Input: part model. Units: mm. Frame: model coordinates. A direction names the side the tool comes from. Coordinates: 2 decimals unless noted, no trailing zeros. Loops run counter-clockwise (first coordinate to the right, second up) from the corner with the lowest first, then second, coordinate; pieces in that order, holes last. Notation, with made-up numbers: M 21,47 L 26,47 A30 cw 26,74 Z; hole C 6.5,51 d11. An arc over 180 degrees is marked long. Use a Markdown table: item, result. Add a question column.
1. Pin query (flat end, axial travel): pin 1 (3 mm diameter, centred on x = 2.5, y = 2, fed in from -Z); pin 2 (2.5 mm diameter, centred on x = 0, y = 0, fed in from -Z); pin 3 (3.5 mm diameter, centred on y = -0.5, z = 13, fed in from +X); pin 4 (8 mm diameter, centred on x = -1.5, y = -20.5, fed in from -Z). Return the tip coordinate at first contact, or that it passes through.
2. Draft query along X for faces 5 (the cylindrical face through (0.29, 2.23, 3.38)), 6 (the flat face through (0, -6, 0)), 7 (the flat face through (-40, 1, -23)). Return one class per face: +X half, -X half, draft (parallel to the pull), parting line (faces both ways), or undercut.
3. Line query: L1, parallel to Y at x = 0, z = 3; L2, parallel to Y at x = -31.5, z = -24; L3, parallel to Y at x = 0, z = 1. Output: solid intervals per line, ascending. Write a range as [from, to].
4. Section C-C on y = 15.5. Output: boundary loops of the cut face in (x, z).
5. Section A-A on x = 0. Output: boundary loops of the cut face in (y, z), then the cut area to 3 significant figures.
6. Section D-D on y = 0. Output: boundary loops of the cut face in (x, z).
7. Section B-B on z = -21. Output: boundary loops of the cut face in (x, y).
8. Set-up query: faces 1 (the flat face through (-15, 4.913, 12)), 2 (the flat face through (-10, -5, 12)), 3 (the cylindrical face through (1.08, -4.88, 0.89)), 4 (the cylindrical face through (-37.47, 7.28, -51.98)). Return all of +Z, -Z, +X, -X, +Y, -Y with unobstructed straight access to the full face (end or side cutting, diameter ignored); none if empty.
```python
from build123d import *

# Parameters (mm, degrees)
SKETCH1_R           = 14
BOSS_EXTRUDE1_DEPTH = 10
SKETCH2_R           = 2.25
CUT_EXTRUDE1_DEPTH  = 5
SKETCH3_R           = 5
CUT_EXTRUDE2_DEPTH  = 1.8
SKETCH4_W           = 10
SKETCH4_H           = 10
BOSS_EXTRUDE2_DEPTH = 8
SKETCH6_W           = 8
SKETCH6_H           = 9.912865289
BOSS_EXTRUDE3_DEPTH = 20
CUT_EXTRUDE3_DEPTH  = 30
SKETCH8_R           = 38
BOSS_EXTRUDE4_DEPTH = 10
SKETCH9_R           = 29
BOSS_EXTRUDE5_DEPTH = 5


with BuildPart() as part:
    # Sketch1 → Boss-Extrude1 (new body)
    with BuildSketch(Plane.XY):
        Circle(SKETCH1_R)
    extrude(amount=BOSS_EXTRUDE1_DEPTH)

    # Sketch2 → Cut-Extrude1 (cut)
    with BuildSketch(Plane(origin=(0, 0, 0), x_dir=(-1, 0, 0), z_dir=(0, 0, -1))):
        Circle(SKETCH2_R)
    extrude(amount=-CUT_EXTRUDE1_DEPTH, mode=Mode.SUBTRACT)

    # Sketch3 → Cut-Extrude2 (cut)
    with BuildSketch(Plane(origin=(0, 0, 0), x_dir=(-1, 0, 0), z_dir=(0, 0, -1))):
        Circle(SKETCH3_R)
    extrude(amount=-CUT_EXTRUDE2_DEPTH, mode=Mode.SUBTRACT)

    # Sketch4 → Boss-Extrude2 (add)
    with BuildSketch(Plane.XY.offset(10)):
        Rectangle(SKETCH4_W, SKETCH4_H)
    extrude(amount=BOSS_EXTRUDE2_DEPTH)

    # Sketch6 → Boss-Extrude3 (add)
    with BuildSketch(Plane.ZY.offset(5)):
        with Locations((14, -0.043567356)):
            Rectangle(SKETCH6_W, SKETCH6_H)
    extrude(amount=BOSS_EXTRUDE3_DEPTH)

    # Sketch7 → Cut-Extrude3 (cut)
    with BuildSketch(Plane(origin=(5, 0, 0), x_dir=(0, 0, -1), z_dir=(1, 0, 0))):
        with BuildLine():
            Line((-18, 5), (-18, -5))
            Line((-18, -5), (-14, -5))
            ThreePointArc((-14, -5), (-14.330383596, 0), (-14, 5))
            Line((-14, 5), (-18, 5))
        make_face()
    extrude(amount=-CUT_EXTRUDE3_DEPTH, mode=Mode.SUBTRACT)

    # Sketch8 → Boss-Extrude4 (add)
    with BuildSketch(Plane.ZY.offset(25)):
        with Locations(Location((-23.669616404, 0, 0), (0, 0, 7.560843177))):
            Circle(SKETCH8_R)
    extrude(amount=BOSS_EXTRUDE4_DEPTH)

    # Sketch9 → Boss-Extrude5 (add)
    with BuildSketch(Plane.ZY.offset(35)):
        with Locations(Location((-23.669616404, 0.99287457, 0), (0, 0, 270))):
            Circle(SKETCH9_R)
    extrude(amount=BOSS_EXTRUDE5_DEPTH)


solid = part.part
```
Answers below:
| question | item | result |
|---|---|---|
| 1 | pin 1 | stops at z = 1.8 |
| 1 | pin 2 | stops at z = 5 |
| 1 | pin 3 | stops at x = 5 |
| 1 | pin 4 | passes through |
| 2 | face 5 | undercut |
| 2 | face 6 | draft |
| 2 | face 7 | -X half |
| 3 | L1 | y = [-14, -2.25], [2.25, 14] |
| 3 | L2 | y = [-38, 38] |
| 3 | L3 | y = [-14, -5], [5, 14] |
| 4 | outline | M -40,-48.78 L -35,-48.78 L -35,-58.36 L -25,-58.36 L -25,11.03 L -35,11.03 L -35,1.44 L -40,1.44 Z |
| 5 | outline | M -14,0 L -5,0 L -5,1.8 L -2.25,1.8 L -2.25,5 L 2.25,5 L 2.25,1.8 L 5,1.8 L 5,0 L 14,0 L 14,10 L 5,10 L 5,14 A38 ccw -5,14 L -5,10 L -14,10 Z |
| 5 | area | 290 mm² |
| 6 | outline | M -40,-52.65 L -35,-52.65 L -35,-61.67 L -25,-61.67 L -25,10 L -14,10 L -14,0 L -5,0 L -5,1.8 L -2.25,1.8 L -2.25,5 L 2.25,5 L 2.25,1.8 L 5,1.8 L 5,0 L 14,0 L 14,10 L 5,10 L 5,14.33 L -35,14.33 L -35,5.31 L -40,5.31 Z |
| 7 | outline | M -40,-27.88 L -35,-27.88 L -35,-37.91 L -25,-37.91 L -25,37.91 L -35,37.91 L -35,29.87 L -40,29.87 Z |
| 8 | face 1 | +Z, +Y |
| 8 | face 2 | +Z, +X, -Y |
| 8 | face 3 | -Z |
| 8 | face 4 | -X |
